The drawing under review shows one solid part. Ordinate dimensions are in mm from its lowest x, y, z. A direction names the side the tool comes from. Round coordinates to 2 decimals unless told otherwise and drop trailing zeros. Order: outer loops, then holes, each group sorted by start corner. A loop starts at its lowest first (then second) coordinate and runs counter-clockwise, first axis right, second up.
1) Consider section A-A (z = 6.25). Give the boundary of the cut face in (x, y).
2) To check wall thickness, follow L1, parallel to Z at x = 7, y = 11.8; L2, parallel to Y at x = 7, z = 17; L3, parallel to Z at x = 8, y = 2.5. State the ranges of each line that lie inside material, in increasing order.
3) Clearance check with flat-ended pins moving along their axes: P1, Ø1.4, axis at x = 6.5, z = 3.5, coming from the -Y side; P2, Ø1.5, axis at x = 10.5, y = 2, coming from the -Z side; P3, Ø1.5, axis at y = 5, z = 4.5, coming from the -X side. State where each tip first meets the part, or that it passes through.
4) Mouldability with a two-part tool opening along X and no side actions: class the marked faces 4, 5, 6 and 7 as pulls with the +X half, pulls with the -X half, needs draft (parallel to the pull), parting line crosses it, or undercut.
5) Machinability: for the marked faces 1, 2 and 3, which of the approach directions +Z, -Z, +X, -X, +Y, -Y give a long, thin tool a straight path to every point of the face, cutting with its end or side? Answer none if there is none.
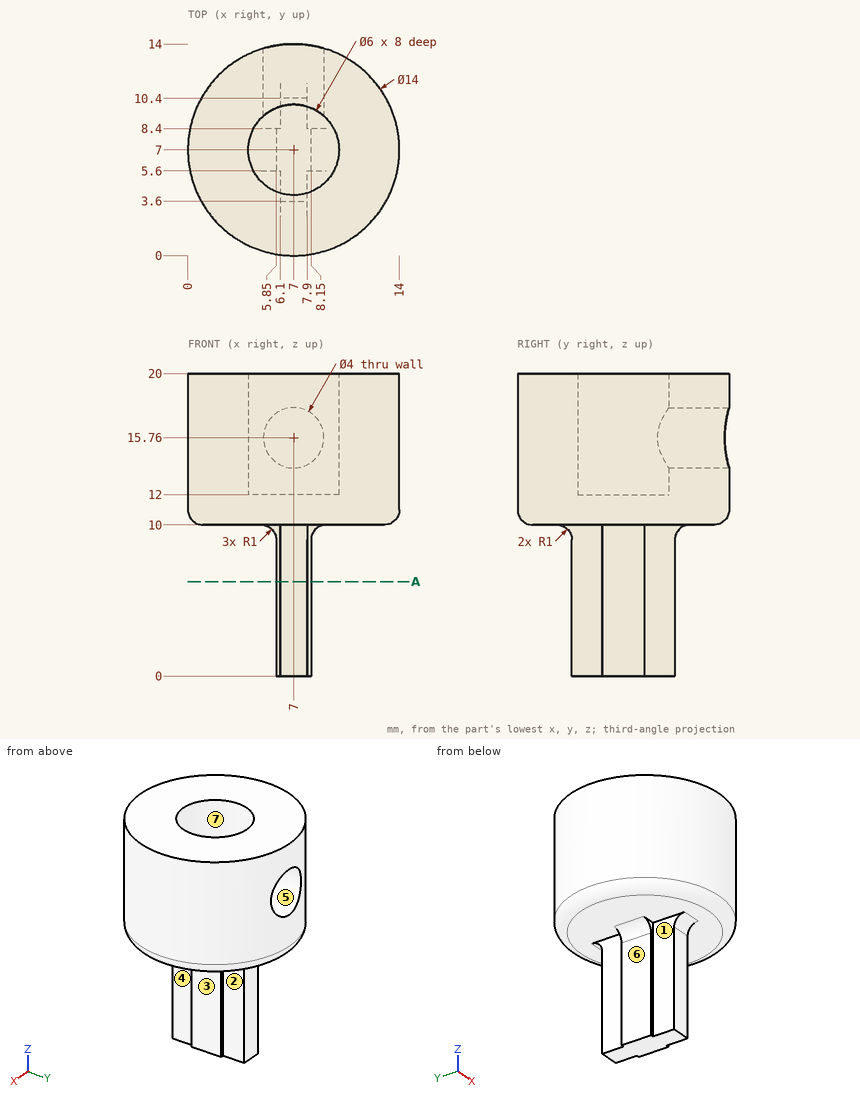
Answer below:
1. outline: (5.85, 5.6) - (6.1, 5.6) - (6.1, 3.6) - (7.9, 3.6) - (7.9, 5.6) - (8.15, 5.6) - (8.15, 8.4) - (7.9, 8.4) - (7.9, 10.4) - (6.1, 10.4) - (6.1, 8.4) - (5.85, 8.4) - close
2. L1: z = 10 to 13.76, 17.76 to 20
2. L2: y = 0 to 4
2. L3: z = 10 to 20
3. P1: stops at y = 3.6
3. P2: stops at z = 10
3. P3: stops at x = 5.85
4. face 4: pulls with the +X half
4. face 5: undercut
4. face 6: pulls with the -X half
4. face 7: undercut
5. face 1: -Z, -X, -Y
5. face 2: -Z, +X, +Y
5. face 3: -Z, +X, +Y, -Y
